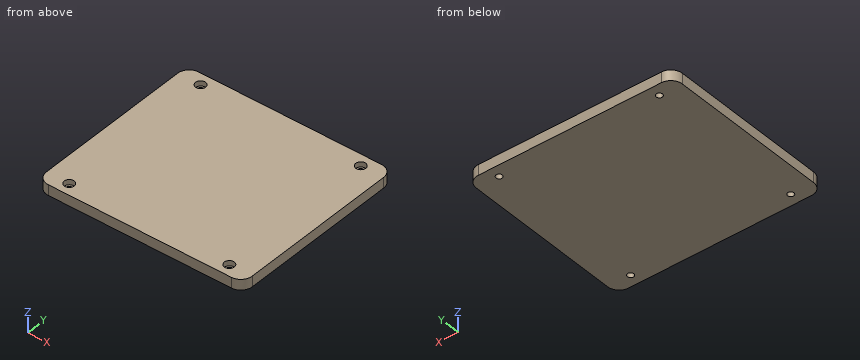
from build123d import *

# Parameters (mm, degrees)
SKETCH1_W                                      = 114.3
SKETCH1_H                                      = 101.6
BOSS_EXTRUDE1_DEPTH                            = 5.842
CBORE_FOR_4_SOCKET_HEAD_CAP_SCREW1_D           = 3.4544
CBORE_FOR_4_SOCKET_HEAD_CAP_SCREW1_CBORE_D     = 5.55752
CBORE_FOR_4_SOCKET_HEAD_CAP_SCREW1_CBORE_DEPTH = 2.8448
FILLET1_R                                      = 6.35


with BuildPart() as part:
    # Sketch1 → Boss-Extrude1 (new body)
    with BuildSketch(Plane.XY):
        Rectangle(SKETCH1_W, SKETCH1_H)
    extrude(amount=BOSS_EXTRUDE1_DEPTH)

    # CBORE for #4 Socket Head Cap Screw1 (through all)
    with Locations(Plane.XY.offset(5.842)):
        with Locations((-44.45, 44.45), (-44.45, -44.45), (44.45, -44.45), (44.45, 44.45)):
            CounterBoreHole(CBORE_FOR_4_SOCKET_HEAD_CAP_SCREW1_D / 2, CBORE_FOR_4_SOCKET_HEAD_CAP_SCREW1_CBORE_D / 2, CBORE_FOR_4_SOCKET_HEAD_CAP_SCREW1_CBORE_DEPTH)

    # Fillet1
    fillet1_edges = [part.edges().sort_by_distance(p)[0] for p in [
        (57.15, -50.8, 2.921),
        (-57.15, -50.8, 2.921),
        (-57.15, 50.8, 2.921),
        (57.15, 50.8, 2.921),
    ]]
    fillet(fillet1_edges, radius=FILLET1_R)


solid = part.part
The model under review builds one solid part; all positions refer to its coordinate system, in mm. Give positions to 0.01 mm unless a question says otherwise; leave off trailing zeros. Order: outer loops, then holes, each group sorted by start corner. A loop starts at its lowest first (then second) coordinate and runs counter-clockwise, first axis right, second up. Notation, with made-up numbers: (22, -14) -> (66, -14) arc R15 ccw to (66, 15) -> close; hole circle Ø1 at (-40, -22.5). An arc over 180 degrees is marked (long way). Write item = value, one per line. Start each with the question number.
(1) For L1, parallel to Y at x = -44.45, z = 2.15; L2, parallel to Y at x = 44.45, z = 4.4; L3, parallel to X at y = -45, z = 4.2, list the stretches that pass through material, from the lowest coordinate up. Write a range as from..to.
(2) Take a section at A-A (x = -44.45). Write out the cut boundary in (y, z), plus the area to 3 significant figures.
(3) For pin 1 Ø3 at (x, y) = (44, 44.5) entering from +Z; pin 2 Ø3 at (x, y) = (44.45, -44.45) entering from +Z; pin 3 Ø1 at (x, y) = (43.5, -21.5) entering from -Z, all flat-tipped, find the tip position at first contact; note any pin that passes through.
Returned:
q1.L1 = -50.8..-46.18, -42.72..42.72, 46.18..50.8
q1.L2 = -50.8..-47.23, -41.67..41.67, 47.23..50.8
q1.L3 = -57.13..-47.17, -41.73..41.73, 47.17..57.13
q2.outline = (-50.8, 0) -> (-46.18, 0) -> (-46.18, 3) -> (-47.23, 3) -> (-47.23, 5.84) -> (-50.8, 5.84) -> close; (-42.72, 0) -> (42.72, 0) -> (42.72, 3) -> (41.67, 3) -> (41.67, 5.84) -> (-41.67, 5.84) -> (-41.67, 3) -> (-42.72, 3) -> close; (46.18, 0) -> (50.8, 0) -> (50.8, 5.84) -> (47.23, 5.84) -> (47.23, 3) -> (46.18, 3) -> close
q2.area = 541 mm²
q3.pin_1 = 3
q3.pin_2 = through
q3.pin_3 = 0
